The model under review builds one solid part; all positions refer to its coordinate system, in mm. Face numbers are marked on the shaded views. Coordinates: 2 decimals unless noted, no trailing zeros. Loops run counter-clockwise (first coordinate to the right, second up) from the corner with the lowest first, then second, coordinate; pieces in that order, holes last. Notation, with made-up numbers: M 82.5,54 L 130.5,54 A27 ccw 130.5,84 Z; hole C 60.5,58.25 d3. An arc over 180 degrees is marked long. Use CSV: the item, a comma, the result in double quotes. Start each with the question number.
1. Add section D-D, the plane y = 1. Write out the cut boundary in (x, z).
2. For L1, parallel to Y at x = -25, z = 5.5; L2, parallel to Y at x = -45, z = 4.5; L3, parallel to X at y = -7.5, z = 2.25, list the stretches that pass through material, from the lowest coordinate up.
3. Add section C-C, the plane y = -13. Write out the cut boundary in (x, z), then the cut area to 3 significant figures.
4. Draft analysis for pull direction X (two halves, no side actions). For the marked faces 1, 2 and 3, state which applies: +X half, -X half, draft (parallel to the pull), parting line (faces both ways), or undercut.
5. Clearance check with flat-ended pins moving along their axes: P1, Ø10, axis at x = -15, y = 15.5, coming from the -Z side; P2, Ø18, axis at x = -25, y = 0, coming from the -Z side. State where each tip first meets the part, or that it passes through.
6. Add section B-B, the plane z = 7. Write out the cut boundary in (x, y).
7. Add section A-A, the plane x = -25. Write out the cut boundary in (y, z).
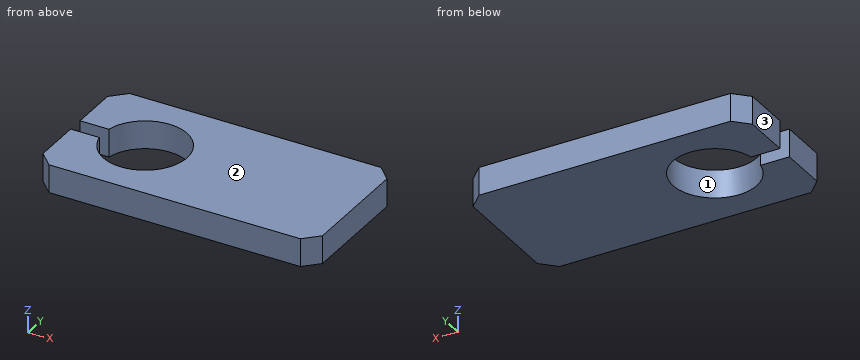
from build123d import *

# Parameters (mm, degrees)
F0_W     = 100
F0_H     = 50
F1_DEPTH = 10
F3_DEPTH = 25
F4_SIZE  = 5


with BuildPart() as f1:
    # F0 (on Top) → F1 (new body)
    with BuildSketch(Plane.XY):
        Rectangle(F0_W, F0_H)
    extrude(amount=F1_DEPTH)

    # F2 (on face) → F3 (cut)
    with BuildSketch(Plane.XY.offset(10)):
        with BuildLine():
            Line((-50, -2.854646), (-39.725862, -2.854646))
            ThreePointArc((-39.725862, -2.854646), (-10.000128, -0.062081), (-39.701728, 2.97644))
            Line((-39.701728, 2.97644), (-50, 2.97644))
            Line((-50, 2.97644), (-50, -2.854646))
        make_face()
    extrude(amount=-F3_DEPTH, mode=Mode.SUBTRACT)

    # F4
    f4_edges = [f1.edges().sort_by_distance(p)[0] for p in [
        (50, 25, 5),
        (50, -25, 5),
        (-50, 25, 5),
        (-50, -25, 5),
    ]]
    chamfer(f4_edges, length=F4_SIZE)


solid = f1.part
Computed:
1,outline,"M -10.03,0 L 50,0 L 50,10 L -10.03,10 Z"
2,L1,"y = -25 to -15, 15 to 25"
2,L2,"y = -25 to -2.85, 2.98 to 25"
2,L3,"x = -50 to -37.99, -12.01 to 50"
3,outline,"M -50,0 L -32.48,0 L -32.48,10 L -50,10 Z; M -17.52,0 L 50,0 L 50,10 L -17.52,10 Z"
3,area,"850 mm^2"
4,face 1,"undercut"
4,face 2,"draft"
4,face 3,"-X half"
5,P1,"stops at z = 0"
5,P2,"passes through"
6,outline,"M -50,-20 L -45,-25 L 45,-25 L 50,-20 L 50,20 L 45,25 L -45,25 L -50,20 L -50,2.98 L -39.7,2.98 A15 cw long -39.73,-2.85 L -50,-2.85 Z"
7,outline,"M -25,0 L -15,0 L -15,10 L -25,10 Z; M 15,0 L 25,0 L 25,10 L 15,10 Z"
